Study the drawing (mm; zero at the part's minimum x, y, z) and answer. Give positions to 0.01 mm unless a question says otherwise; leave off trailing zeros. Order: outer loops, then holes, each group sorted by start corner. A loop starts at its lowest first (then second) coordinate and runs counter-clockwise, first axis right, second up.
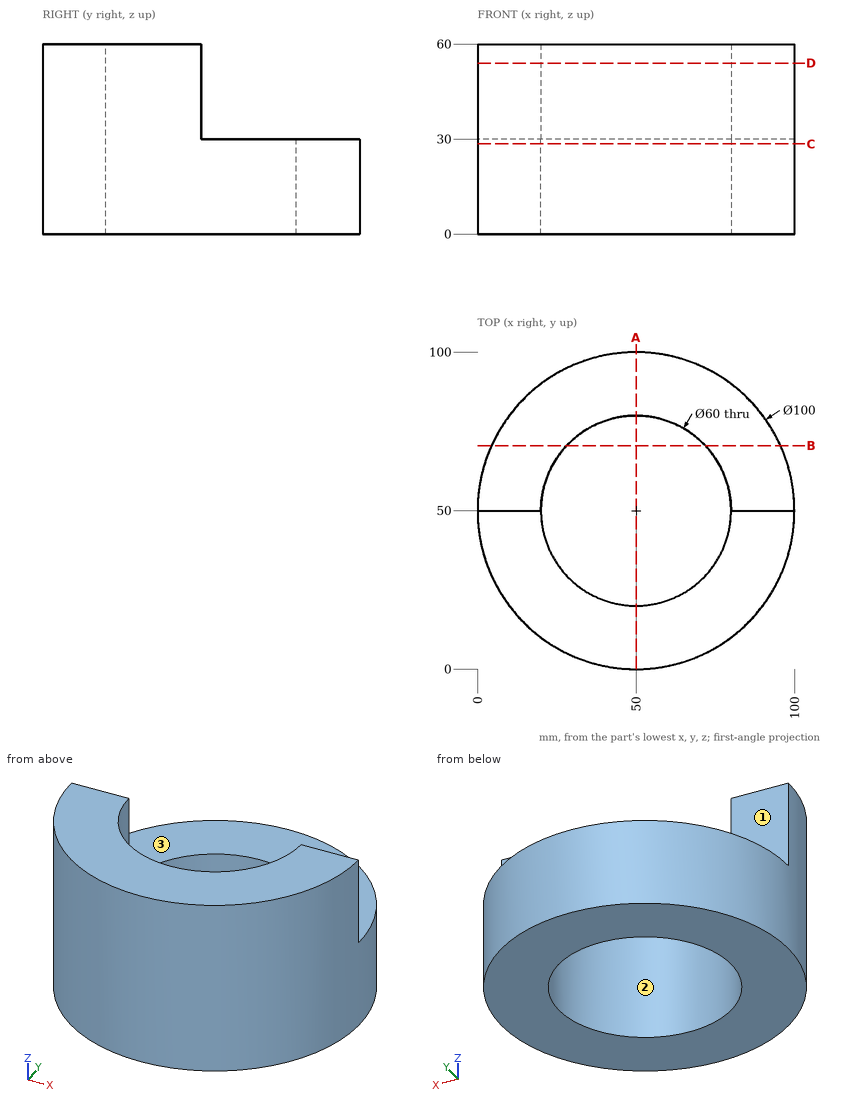
1) Given P1, Ø10, axis at y = 77, z = 7.5, coming from the +X side; P2, Ø12, axis at x = 87, z = 47, coming from the +Y side; P3, Ø2, axis at x = 45, z = 51, coming from the -Y side, each flat-ended and moving along its own axis, determine where each tip first touches the part or whether it passes through.
Geometry says:
P1: stops at x = 94.9
P2: stops at y = 50
P3: stops at y = 0.16
2) Find section D-D (z = 54). Write down the section's boundary in (x, y).
Geometry says:
outline: (0, 50) arc R50 ccw to (100, 50) - (80, 50) arc R30 cw to (20, 50) - close
3) Straight lines are drawn through the part: probe 1 along Y at (x, z) = (50, 16); probe 2 along Y at (x, z) = (22.5, 16.5); probe 3 along Z at (x, y) = (58.5, 91). For each, find the intervals that lie inside material, in ascending order.
Geometry says:
probe 1: y = 0 to 20, 80 to 100
probe 2: y = 8.24 to 38.01, 61.99 to 91.76
probe 3: z = 0 to 30
4) Find section A-A (x = 50). Write down the section's boundary in (y, z).
Geometry says:
outline: (0, 0) - (20, 0) - (20, 60) - (0, 60) - close; (80, 0) - (100, 0) - (100, 30) - (80, 30) - close
5) Find section B-B (y = 70.5). Write down the section's boundary in (x, z).
Geometry says:
outline: (4.4, 0) - (28.1, 0) - (28.1, 30) - (4.4, 30) - close; (71.9, 0) - (95.6, 0) - (95.6, 30) - (71.9, 30) - close
6) For a pull along Y with two mould halves and no side action, classify the marked faces 1, 2 and 3 as +Y half, -Y half, draft (parallel to the pull), parting line (faces both ways), or undercut.
Geometry says:
face 1: +Y half
face 2: undercut
face 3: draft
7) Find section C-C (z = 28.5). Write down the section's boundary in (x, y).
Geometry says:
outline: circle Ø100 at (50, 50); hole circle Ø60 at (50, 50)
